from build123d import *

# Parameters (mm, degrees)
F0_W          = 1
F0_H          = 8
F2_ANGLE_BACK = 9.5
F2_ANGLE      = 19


with BuildPart() as f1:
    # F0 (on Front) → F1 (revolve)
    with BuildSketch(Plane.XZ):
        Polygon((48.960784, 2.9816715978), (48.960784, 0), (50.960784, 0), (50.960784, 1), (49.960784, 1), (49.960784, 2.9816715978), align=None)
        with Locations((49.460784, 6.9816715978)):
            Rectangle(F0_W, F0_H)
    revolve(axis=Axis((0, 0, 8.8810138404), (0, 0, 1)))

    # F0 (on Front) → F2 (revolve, cut)
    with BuildSketch(Plane.XZ, mode=Mode.PRIVATE) as f2_sk:
        with Locations((49.460784, 6.9816715978)):
            Rectangle(F0_W, F0_H)
    revolve(f2_sk.sketch.rotate(Axis((0, 0, 8.8810138404), (0, 0, 1)), -F2_ANGLE_BACK), axis=Axis((0, 0, 8.8810138404), (0, 0, 1)), revolution_arc=F2_ANGLE, mode=Mode.SUBTRACT)


solid = f1.part
Input: part model. Units: mm. Frame: model coordinates. A direction names the side the tool comes from. Coordinates: 2 decimals unless noted, no trailing zeros. Order: outer loops, then holes, each group sorted by start corner. A loop starts at its lowest first (then second) coordinate and runs counter-clockwise, first axis right, second up.
1. Cut plane A-A, the plane y = 0. Return loops of the section in (x, z), plus the area to 3 significant figures.
Checked values:
outline: (-50.96, 0) - (-48.96, 0) - (-48.96, 10.98) - (-49.96, 10.98) - (-49.96, 1) - (-50.96, 1) - close; (48.96, 0) - (50.96, 0) - (50.96, 1) - (49.96, 1) - (49.96, 2.98) - (48.96, 2.98) - close
area: 16.0 mm2
2. Cut plane C-C, the plane z = 4.5. Return loops of the section in (x, y).
Checked values:
outline: (48.29, -8.08) arc R48.96 cw (long way) to (48.29, 8.08) - (49.28, 8.25) arc R49.96 ccw (long way) to (49.28, -8.25) - close
3. Cut plane B-B, the plane x = 0. Return loops of the section in (y, z), plus the area to 3 significant figures.
Checked values:
outline: (-50.96, 0) - (-48.96, 0) - (-48.96, 10.98) - (-49.96, 10.98) - (-49.96, 1) - (-50.96, 1) - close; (48.96, 0) - (50.96, 0) - (50.96, 1) - (49.96, 1) - (49.96, 10.98) - (48.96, 10.98) - close
area: 24.0 mm2
4. Draft query along Y for faces 1 (the flat face through (19, 46, 0)), 2 (the cylindrical face through (-11.05, -49.75, 0.51)), 3 (the cylindrical face through (46.7, 14.7, 5.4)). Return one class per face: +Y half, -Y half, draft (parallel to the pull), parting line (faces both ways), or undercut.
Checked values:
face 1: draft
face 2: parting line
face 3: undercut
5. Contact query for flat-ended pins moving along their axis: P1, Ø1, axis at x = 35, z = 2, coming from the +Y side; P2, Ø0.5, axis at x = 49.5, y = -3.5, coming from the +Z side; P3, Ø5, axis at x = 9.5, z = 8, coming from the -Y side. Output: stop coordinate, or through.
Checked values:
P1: stops at y = 36.14
P2: stops at z = 2.98
P3: stops at y = -49.47
6. Ray query, line 1 along Y through (x, z) = (0, 5); line 2 along X through (y, z) = (-26, 9.75); line 3 along X through (y, z) = (0, 7.5). Return the intervals inside material, ascending.
Checked values:
line 1: y = -49.96 to -48.96, 48.96 to 49.96
line 2: x = -42.66 to -41.49, 41.49 to 42.66
line 3: x = -49.96 to -48.96
7. Access query for faces 4 (the cylindrical face through (46.15, -19.14, 6.06)), 5 (the flat face through (44, -22, 10.982)). Directions: +Z, -Z, +X, -X, +Y, -Y. A direction counts if a zero-diameter tool reaches every point of the face in a straight line with its end or side. Return the directions, or none.
Checked values:
face 4: +Z
face 5: +Z, +X, -X, +Y, -Y
